from build123d import *

# Parameters (mm, degrees)
SKETCH2_R             = 85.5
BOSS_EXTRUDE1_DEPTH   = 5
SKETCH4_R             = 75.5
BOSS_EXTRUDE2_DEPTH   = 28
SKETCH5_R             = 29
CUT_EXTRUDE1_DEPTH    = 126.337544256
CUT_EXTRUDE2_DEPTH    = 126.337544256
CIRPATTERN1_COUNT     = 5
SKETCH10_R            = 3
CUT_EXTRUDE3_DEPTH    = 12
CIRPATTERN2_COUNT     = 2
CIRPATTERN2_ANGLE     = 60
CIRPATTERN3_START     = 21
CIRPATTERN3_OUTLINE_R = 3
CIRPATTERN3_DEPTH     = 12


# Read off the part's stored shape, not the designer's step: CirPattern3
with BuildPart() as part:
    # Sketch2 → Boss-Extrude1 (new body)
    with BuildSketch(Plane.XY):
        Circle(SKETCH2_R)
    extrude(amount=BOSS_EXTRUDE1_DEPTH)

    # Sketch4 → Boss-Extrude2 (add)
    with BuildSketch(Plane.XY.offset(5)):
        Circle(SKETCH4_R)
    extrude(amount=BOSS_EXTRUDE2_DEPTH)

    # Sketch5 → Cut-Extrude1 (cut, through all)
    with BuildSketch(Plane.XY.offset(33)):
        with Locations((0, -23)):
            Circle(SKETCH5_R)
    extrude(amount=-CUT_EXTRUDE1_DEPTH, mode=Mode.SUBTRACT)

    # Sketch7 → Cut-Extrude2 (cut, symmetric)
    with BuildSketch(Plane.XY.offset(33)):
        with BuildLine():
            Line((-7, 8.737202145), (-7, 5.142494559))
            ThreePointArc((-7, 5.142494559), (0, 6), (7, 5.142494559))
            Line((7, 5.142494559), (7, 8.737202145))
            ThreePointArc((7, 8.737202145), (0, 9.5), (-7, 8.737202145))
        make_face()
    cut_extrude2 = extrude(amount=CUT_EXTRUDE2_DEPTH, both=True, mode=Mode.SUBTRACT)

    # CirPattern1: Cut-Extrude2 ×5 about axis
    cirpattern1_axis = Axis((0, -23, 0), (0, 0, 1))
    for i in range(1, CIRPATTERN1_COUNT):
        add(cut_extrude2.rotate(cirpattern1_axis, i * 360 / CIRPATTERN1_COUNT), mode=Mode.SUBTRACT)

    # Sketch10 → Cut-Extrude3 (cut)
    with BuildSketch(Plane.XY.offset(33)):
        with Locations((0, 67)):
            Circle(SKETCH10_R)
    cut_extrude3 = extrude(amount=-CUT_EXTRUDE3_DEPTH, mode=Mode.SUBTRACT)

    # CirPattern2: Cut-Extrude3 ×2 about axis
    cirpattern2_axis = Axis((0, 0, 5), (0, 0, 1))
    for i in range(1, CIRPATTERN2_COUNT):
        add(cut_extrude3.rotate(cirpattern2_axis, i * CIRPATTERN2_ANGLE / (CIRPATTERN2_COUNT - 1)), mode=Mode.SUBTRACT)

    # CirPattern3 outline → CirPattern3 (cut)
    with BuildSketch(Plane.XY.offset(CIRPATTERN3_START)):
        with Locations((58.023702054, 33.5)):
            Circle(CIRPATTERN3_OUTLINE_R)
    extrude(amount=CIRPATTERN3_DEPTH, mode=Mode.SUBTRACT)


solid = part.part
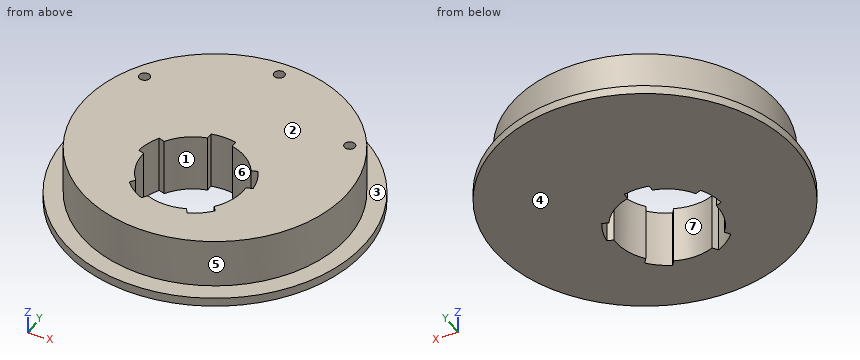
Read the model definition and answer for the solid it produces. Units are mm, in the model's axes. Face numbers are marked on the shaded views. A direction names the side the tool comes from. Coordinates: 2 decimals unless noted, no trailing zeros. Loops run counter-clockwise (first coordinate to the right, second up) from the corner with the lowest first, then second, coordinate; pieces in that order, holes last.
Q1. The mould has two halves that part along X. Classify the marked faces 4, 5, 6 and 7: +X half, -X half, draft (parallel to the pull), parting line (faces both ways), or undercut.
Q2. The part is cut by section B-B on z = 9. Write down the section's boundary in (x, y), and give its area (3 significant figures).
Q3. The part is cut by section C-C on y = 0. Write down the section's boundary in (x, z).
Q4. The part is cut by section D-D on x = -41. Write down the section's boundary in (y, z).
Q5. Each of these flat-tipped pins is pushed along its axis until it touches: pin 1 Ø4 at (y, z) = (6.5, 9.5) entering from -X; pin 2 Ø5 at (x, y) = (31.5, 54) entering from -Z; pin 3 Ø1.8 at (x, y) = (0, 68) entering from +Z; pin 4 Ø12 at (y, z) = (54.5, 27) entering from +X. Where does it stop, or does it pass through?
Q6. Which of the six approach directions +Z, -Z, +X, -X, +Y, -Y give full straight-line access (tool end or side, diameter ignored) to the marked faces 1, 2 and 3?
Q7. The part is cut by section A-A on x = 0. Write down the section's boundary in (y, z), and give its area (3 significant figures).
Q8. Consider probe 1 along Y at (x, z) = (-23, 25); probe 2 along Y at (x, z) = (-21.5, 10.5); probe 3 along X at (y, z) = (-22.5, 8). Determine where each line is inside the solid, lowest interval first.
Results below:
1. face 4: draft
1. face 5: parting line
1. face 6: undercut
1. face 7: undercut
2. outline: circle Ø151 at (0, 0); hole (-32.35, -19.85) - (-28.93, -20.96) arc R29 ccw to (-22.2, -41.65) - (-24.32, -44.56) arc R32.5 ccw to (-12.99, -52.79) - (-10.88, -49.88) arc R29 ccw to (10.88, -49.88) - (12.99, -52.79) arc R32.5 ccw to (24.32, -44.56) - (22.2, -41.65) arc R29 ccw to (28.93, -20.96) - (32.35, -19.85) arc R32.5 ccw to (28.02, -6.54) - (24.6, -7.65) arc R29 ccw to (7, 5.14) - (7, 8.74) arc R32.5 ccw to (-7, 8.74) - (-7, 5.14) arc R29 ccw to (-24.6, -7.65) - (-28.02, -6.54) arc R32.5 ccw to start
2. area: 15,000 mm2
3. outline: (-85.5, 0) - (-17.66, 0) - (-17.66, 33) - (-75.5, 33) - (-75.5, 5) - (-85.5, 5) - close; (17.66, 0) - (85.5, 0) - (85.5, 5) - (75.5, 5) - (75.5, 33) - (17.66, 33) - close
4. outline: (-75.03, 0) - (75.03, 0) - (75.03, 5) - (63.4, 5) - (63.4, 33) - (-63.4, 33) - (-63.4, 5) - (-75.03, 5) - close
5. pin 1: stops at x = -75.37
5. pin 2: stops at z = 0
5. pin 3: stops at z = 21
5. pin 4: stops at x = 57.86
6. face 1: +Z, -Z
6. face 2: +Z, +X, -X, +Y, -Y
6. face 3: +Z
7. outline: (-85.5, 0) - (-52, 0) - (-52, 33) - (-75.5, 33) - (-75.5, 5) - (-85.5, 5) - close; (9.5, 0) - (85.5, 0) - (85.5, 5) - (75.5, 5) - (75.5, 33) - (70, 33) - (70, 21) - (64, 21) - (64, 33) - (9.5, 33) - close
7. area: 2,980 mm2
8. probe 1: y = -71.91 to -45.96, -42.75 to -40.66, -5.34 to 71.91
8. probe 2: y = -72.37 to -47.37, -3.54 to 72.37
8. probe 3: x = -72.07 to -29, 29 to 72.07
